```python
from build123d import *

# Parameters (mm, degrees)
ESTRUSIONE_ESTRUSIONE1_DEPTH = 21
ESTRUSIONE_ESTRUSIONE2_DEPTH = 19
FORO_PER_VITE_M6_5_1_D       = 7.1
FORO_PER_VITE_M6_5_1_DEPTH   = 80
FORO_PER_VITE_M6_5_1_TIP     = 2.133055198
SCHIZZO5_R                   = 19
ESTRUSIONE_ESTRUSIONE3_DEPTH = 74
SCHIZZO7_R                   = 6.25
ESTRUSIONE_ESTRUSIONE4_DEPTH = 3.5
ESTRUSIONE_ESTRUSIONE5_DEPTH = 198
ESTRUSIONE_ESTRUSIONE6_DEPTH = 12
SCHIZZO10_R                  = 10
ESTRUSIONE_ESTRUSIONE7_DEPTH = 22
FORO_PER_VITE_M6_1_D         = 6.6
FORO_PER_VITE_M6_1_DEPTH     = 80
FORO_PER_VITE_M6_1_TIP       = 1.982840043


with BuildPart() as part:
    # Schizzo1 → Estrusione-Estrusione1 (new body)
    # profile 1 of 2: a face of its own
    with BuildSketch(Plane(origin=(0, 0, 0), x_dir=(1, 0, 0), z_dir=(0, 1, 0))):
        with BuildLine():
            Line((20, 7), (20, 55))
            ThreePointArc((20, 55), (0, 75), (-20, 55))
            Line((-20, 55), (-20, 7))
            Line((-20, 7), (-11, 0))
            Line((-11, 0), (11, 0))
            Line((11, 0), (20, 7))
        make_face()
        Polygon((9, 24.5), (9, 15.5), (4.5, 11), (-4.5, 11), (-9, 15.5), (-9, 24.5), (-4.5, 29), (4.5, 29), align=None, mode=Mode.SUBTRACT)
    # profile 2 of 2: a face of its own
    with BuildSketch(Plane(origin=(0, 0, 0), x_dir=(1, 0, 0), z_dir=(0, 1, 0))):
        Polygon((9, 15.5), (4.5, 11), (-4.5, 11), (-9, 15.5), (-9, 24.5), (-4.5, 29), (4.5, 29), (9, 24.5), align=None)
    extrude(amount=ESTRUSIONE_ESTRUSIONE1_DEPTH)

    # Schizzo1_3 → Estrusione-Estrusione2 (add)
    with BuildSketch(Plane(origin=(0, 0, 0), x_dir=(1, 0, 0), z_dir=(0, 1, 0))):
        Polygon((9, 15.5), (4.5, 11), (-4.5, 11), (-9, 15.5), (-9, 24.5), (-4.5, 29), (4.5, 29), (9, 24.5), align=None)
    extrude(amount=-ESTRUSIONE_ESTRUSIONE2_DEPTH)

    # Foro per Vite M6.5-1
    with Locations(Plane(origin=(9, 0, 0), x_dir=(0, 0, -1), z_dir=(1, 0, 0))):
        with Locations((20, -9)):
            Hole(FORO_PER_VITE_M6_5_1_D / 2, depth=FORO_PER_VITE_M6_5_1_DEPTH)
            with Locations((0, 0, -(FORO_PER_VITE_M6_5_1_DEPTH + FORO_PER_VITE_M6_5_1_TIP / 2))):  # 118° drill point
                Cone(0, FORO_PER_VITE_M6_5_1_D / 2, FORO_PER_VITE_M6_5_1_TIP, mode=Mode.SUBTRACT)

    # Schizzo5 → Estrusione-Estrusione3 (add)
    with BuildSketch(Plane(origin=(0, 21, 0), x_dir=(1, 0, 0), z_dir=(0, 1, 0))):
        with Locations(Location((0, 55.2, 0), (0, 0, 270))):
            Circle(SCHIZZO5_R)
    extrude(amount=ESTRUSIONE_ESTRUSIONE3_DEPTH)

    # Schizzo7 → Estrusione-Estrusione4 (add)
    with BuildSketch(Plane(origin=(0, 95, 0), x_dir=(1, 0, 0), z_dir=(0, 1, 0))):
        with Locations(Location((0, 55.2, 0), (0, 0, 270))):
            Circle(SCHIZZO7_R)
    extrude(amount=ESTRUSIONE_ESTRUSIONE4_DEPTH)

    # Schizzo8 → Estrusione-Estrusione5 (add)
    with BuildSketch(Plane(origin=(0, 21, 0), x_dir=(1, 0, 0), z_dir=(0, 1, 0))):
        with BuildLine():
            Line((-11, 0), (11, 0))
            Line((11, 0), (14.657188407, 16.811453624))
            ThreePointArc((14.657188407, 16.811453624), (0, 35), (-14.657188407, 16.811453624))
            Line((-14.657188407, 16.811453624), (-11, 0))
        make_face()
    extrude(amount=ESTRUSIONE_ESTRUSIONE5_DEPTH)

    # Schizzo9 → Estrusione-Estrusione6 (add)
    with BuildSketch(Plane(origin=(0, 219, 0), x_dir=(1, 0, 0), z_dir=(0, 1, 0))):
        with BuildLine():
            Line((-12.208770737, -1.5), (12.208770737, -1.5))
            Line((12.208770737, -1.5), (16.192271356, 16.811453624))
            ThreePointArc((16.192271356, 16.811453624), (0, 36.503226341), (-16.192271356, 16.811453624))
            Line((-16.192271356, 16.811453624), (-12.208770737, -1.5))
        make_face()
    extrude(amount=ESTRUSIONE_ESTRUSIONE6_DEPTH)

    # Schizzo10 → Estrusione-Estrusione7 (add)
    with BuildSketch(Plane(origin=(0, 231, 0), x_dir=(1, 0, 0), z_dir=(0, 1, 0))):
        with Locations(Location((0, 20, 0), (0, 0, 270))):
            Circle(SCHIZZO10_R)
    extrude(amount=ESTRUSIONE_ESTRUSIONE7_DEPTH)

    # Foro per Vite M6-1
    with Locations(Plane(origin=(10, 244, -20), x_dir=(0, 0, 1), z_dir=(1, 0, 0))):
        with Locations((0, 0)):
            Hole(FORO_PER_VITE_M6_1_D / 2, depth=FORO_PER_VITE_M6_1_DEPTH)
            with Locations((0, 0, -(FORO_PER_VITE_M6_1_DEPTH + FORO_PER_VITE_M6_1_TIP / 2))):  # 118° drill point
                Cone(0, FORO_PER_VITE_M6_1_D / 2, FORO_PER_VITE_M6_1_TIP, mode=Mode.SUBTRACT)


solid = part.part
```
Verification items for the finished model (mm, model axes). A direction names the side the tool comes from. Round coordinates to 2 decimals unless told otherwise and drop trailing zeros. Order: outer loops, then holes, each group sorted by start corner. A loop starts at its lowest first (then second) coordinate and runs counter-clockwise, first axis right, second up.
1) Cross-section at D-D, the plane y = 69.5. Record the cut outline in (x, z).
Geometry says:
outline: circle Ø38 at (0, -55.2); (-14.66, -16.81) arc R15 ccw (long way) to (14.66, -16.81) - (11, 0) - (-11, 0) - close
2) Cross-section at C-C, the plane z = -59. Record the cut outline in (x, y), plus the area to 3 significant figures.
Geometry says:
outline: (-19.6, 0) - (19.6, 0) - (19.6, 21) - (18.62, 21) - (18.62, 95) - (4.96, 95) - (4.96, 98.5) - (-4.96, 98.5) - (-4.96, 95) - (-18.62, 95) - (-18.62, 21) - (-19.6, 21) - close
area: 3,610 mm2
3) Cross-section at A-A, the plane y = -9. Record the cut outline in (x, z).
Geometry says:
outline: (-9, -24.5) - (-4.5, -29) - (4.5, -29) - (9, -24.5) - (9, -23.55) - (-9, -23.55) - close; (-9, -16.45) - (9, -16.45) - (9, -15.5) - (4.5, -11) - (-4.5, -11) - (-9, -15.5) - close
4) Cross-section at B-B, the plane x = 0. Record the cut outline in (y, z).
Geometry says:
outline: (-19, -29) - (0, -29) - (0, -75) - (21, -75) - (21, -74.2) - (95, -74.2) - (95, -61.45) - (98.5, -61.45) - (98.5, -48.95) - (95, -48.95) - (95, -36.2) - (21, -36.2) - (21, -35) - (219, -35) - (219, -36.5) - (231, -36.5) - (231, -30) - (253, -30) - (253, -10) - (231, -10) - (231, 1.5) - (219, 1.5) - (219, 0) - (0, 0) - (0, -11) - (-19, -11) - close; hole circle Ø7.1 at (-9, -20); hole circle Ø6.6 at (244, -20)
5) Draft check along Y on faces 1 (the flat face through (0, 0, -38)), 2 (the flat face through (-12.854, 118.614, -8.523)), 3 (the flat face through (9, -11.5, -23.1)), 4 (the flat face through (12.803, 118.614, -8.288)). Enter one of: +Y half, -Y half, draft (parallel to the pull), parting line (faces both ways), or undercut.
Geometry says:
face 1: -Y half
face 2: undercut
face 3: draft
face 4: undercut
6) Tool access check on faces 5 (the flat face through (15.437, 10.353, -3.451)), 6 (the cylindrical face through (0.275, 96.726, -61.444)), 7 (the flat face through (0, -9, -11)), 8 (the flat face through (-6.7, -9.4, -13.2)). Record the directions out of +Z, -Z, +X, -X, +Y, -Y that give a thin tool (end or side, any length) a straight path to the whole face; none if there is none.
Geometry says:
face 5: +Z, +X, -Y
face 6: +Y
face 7: +Z, +X, -X, -Y
face 8: +Z, -X, -Y
7) Material ranges on line 1 (Y direction, x = -3.25, z = -20); line 2 (Y direction, x = 16, z = -19); line 3 (Z direction, x = -1, y = 32), recorded low to high.
Geometry says:
line 1: y = -19 to -12.55, -5.45 to 240.7, 247.3 to 253
line 2: y = 0 to 21, 219 to 231
line 3: z = -74.17 to -36.23, -34.97 to 0
8) Depth check by flat-ended pin: pin 1 (7 mm diameter, centred on y = -5, z = -22, fed in from +X); pin 2 (8 mm diameter, centred on x = -13, y = 163, fed in from +Z); pin 3 (19 mm diameter, centred on x = -4, z = -48, fed in from +Y); pin 4 (4.5 mm diameter, centred on y = -9, z = -20, fed in from -X). Enter the tip coordinate at first touch or a pass-through.
Geometry says:
pin 1: stops at x = 9
pin 2: stops at z = 0
pin 3: stops at y = 98.5
pin 4: passes through
